```python
from build123d import *

# Parameters (mm, degrees)
SKETCH1_R      = 1
EXTRUDE1_DEPTH = 1


with BuildPart() as part:
    # Sketch1 → Extrude1 (new body)
    with BuildSketch(Plane.XY):
        with BuildLine():
            ThreePointArc((0, 2), (-2, 0), (0, -2))
            Line((0, -2), (18.16, -2))
            ThreePointArc((18.16, -2), (20.16, 0), (18.16, 2))
            Line((18.16, 2), (0, 2))
        make_face()
        Circle(SKETCH1_R, mode=Mode.SUBTRACT)
        with Locations((18.16, 0)):
            Circle(SKETCH1_R, mode=Mode.SUBTRACT)
    extrude(amount=-EXTRUDE1_DEPTH)


solid = part.part
```
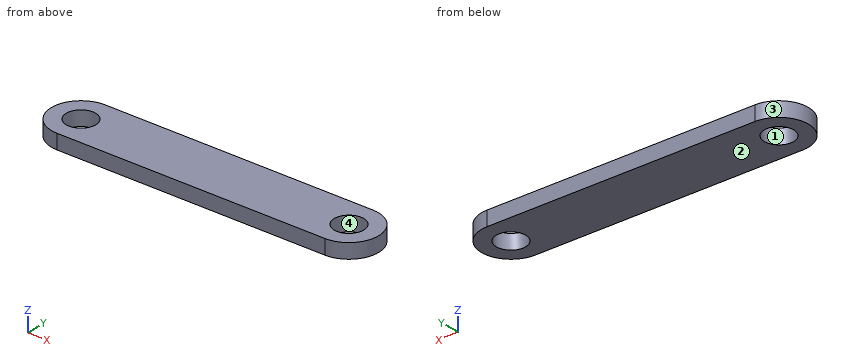
Input: part model. Units: mm. Frame: model coordinates. Face numbers are marked on the shaded views. Coordinates: 2 decimals unless noted, no trailing zeros. Loops run counter-clockwise (first coordinate to the right, second up) from the corner with the lowest first, then second, coordinate; pieces in that order, holes last. Notation, with made-up numbers: M 81.5,6.5 L 135.5,6.5 A13 ccw 135.5,22.5 Z; hole C -20.5,77 d7. An arc over 180 degrees is marked long. One line per item, written item: value.
(1) Section C-C (y = 1.25). Output: boundary loops of the cut face in (x, z).
Filled in:
outline: M -1.56,-1 L 19.72,-1 L 19.72,0 L -1.56,0 Z
(2) Section A-A (y = 0). Output: boundary loops of the cut face in (x, z), and give its area (3 significant figures).
Filled in:
outline: M -2,-1 L -1,-1 L -1,0 L -2,0 Z; M 1,-1 L 17.16,-1 L 17.16,0 L 1,0 Z; M 19.16,-1 L 20.16,-1 L 20.16,0 L 19.16,0 Z
area: 18.2 mm^2
(3) Pull-direction query (X, two-part tool) for the marked faces 1, 2, 3 and 4; classes: +X half, -X half, draft (parallel to the pull), parting line (faces both ways), or undercut.
Filled in:
face 1: undercut
face 2: draft
face 3: -X half
face 4: undercut
(4) Section B-B (z = -0.55). Output: boundary loops of the cut face in (x, y).
Filled in:
outline: M 0,-2 L 18.16,-2 A2 ccw 18.16,2 L 0,2 A2 ccw Z; hole C 0,0 d2; hole C 18.16,0 d2
(5) Pin query (flat end, axial travel): pin 1 (1.2 mm diameter, centred on x = 18.16, y = 0, fed in from -Z) (3 decimals). Return the tip coordinate at first contact, or that it passes through.
Filled in:
pin 1: through
(6) Line query: line 1 along X through (y, z) = (0.05, -0.85); line 2 along Y through (x, z) = (18.16, -0.65); line 3 along X through (y, z) = (0.85, -0.2). Output: solid intervals per line, ascending. Write a range as from..to.
Filled in:
line 1: -2..-1, 1..17.16, 19.16..20.16
line 2: -2..-1, 1..2
line 3: -1.81..-0.53, 0.53..17.63, 18.69..19.97
